Geometry: final body of the model. Coordinates: model frame, mm. A direction names the side the tool comes from. Coordinates: 2 decimals unless noted, no trailing zeros. Write each loop counter-clockwise with the first axis right and the second up, starting at its lowest first coordinate (ties: lowest second). Pieces come first, ordered by that corner, then holes. Notation, with made-up numbers: (70.5, 64) -> (124.5, 64) arc R23 cw to (124.5, 75) -> close; hole circle Ø4 at (51.5, 16). An arc over 180 degrees is marked (long way). One line per item, written item: value.
```python
from build123d import *

# Parameters (mm, degrees)
F3_D = 5.5


with BuildPart() as f1:
    # F0 (on Front) → F1 (revolve)
    with BuildSketch(Plane.XZ):
        Polygon((4, 32.5), (0, 32.5), (0, 23.5), (-2, 23.5), (-2, 18.5), (4, 18.5), align=None)
    revolve(axis=Axis((1.6395361068, 0, 0), (1, 0, 0)))

    # F3 (through all)
    with Locations(Plane(origin=(0, 0, 0), x_dir=(0, -1, 0), z_dir=(-1, 0, 0))):
        with Locations((0, 28), (28, 0), (0, -28), (-28, 0)):
            Hole(F3_D / 2)


solid = f1.part
```
(1) Line query: line 1 (Z direction, x = 2.75, y = 0); line 2 (Y direction, x = 2.2, z = 2); line 3 (X direction, y = -29, z = -6.5). Output: solid intervals per line, ascending. Write a range as [from, to].
Responses:
line 1: z = [-32.5, -30.75], [-25.25, -18.5], [18.5, 25.25], [30.75, 32.5]
line 2: y = [-32.44, -29.89], [-26.11, -18.39], [18.39, 26.11], [29.89, 32.44]
line 3: x = [0, 4]
(2) Pull-direction query (Y, two-part tool) for faces 1 (the cylindrical face through (-1, -7.1, 22.4)), 2 (the flat face through (4, 14, -14)), 3 (the cylindrical face through (2.028, -0.358, 30.727)), 4 (the cylindrical face through (2.028, 25.253, 0.121)); classes: released by +Y, released by -Y, zero draft, split by the parting line, or undercut.
Responses:
face 1: split by the parting line
face 2: zero draft
face 3: undercut
face 4: undercut
(3) Section A-A (z = 0). Return the cut outline in (x, y), then the cut area to 3 significant figures.
Responses:
outline: (-2, -23.5) -> (0, -23.5) -> (0, -25.25) -> (4, -25.25) -> (4, -18.5) -> (-2, -18.5) -> close; (-2, 18.5) -> (4, 18.5) -> (4, 25.25) -> (0, 25.25) -> (0, 23.5) -> (-2, 23.5) -> close; (0, -32.5) -> (4, -32.5) -> (4, -30.75) -> (0, -30.75) -> close; (0, 30.75) -> (4, 30.75) -> (4, 32.5) -> (0, 32.5) -> close
area: 88.0 mm2
(4) Reachability of faces 5 (the cylindrical face through (1.04, 18.06, -4.01)), 6 (the flat face through (0, 9, 22)) from +Z, -Z, +X, -X, +Y, -Y: full face, straight path, thin tool, end or side. Return the list, or none.
Responses:
face 5: +X, -X
face 6: -X
(5) First-contact query: pin 1 (7 mm diameter, centred on y = -28, z = 0, fed in from -X); pin 2 (5 mm diameter, centred on y = 0, z = 28, fed in from +X); pin 3 (3 mm diameter, centred on x = 2.5, y = 20, fed in from +Z). Flat tips, straight axial feed; report the tip coordinate or a pass-through.
Responses:
pin 1: stops at x = 0
pin 2: passes through
pin 3: stops at z = 26.72
(6) Section C-C (y = 28). Return the cut outline in (x, z).
Responses:
outline: (0, -16.5) -> (4, -16.5) -> (4, -2.75) -> (0, -2.75) -> close; (0, 2.75) -> (4, 2.75) -> (4, 16.5) -> (0, 16.5) -> close
(7) Section D-D (x = 2.15). Return the cut outline in (y, z), then the cut area to 3 significant figures.
Responses:
outline: circle Ø65 at (0, 0); hole circle Ø5.5 at (-28, 0); hole circle Ø37 at (0, 0); hole circle Ø5.5 at (0, -28); hole circle Ø5.5 at (0, 28); hole circle Ø5.5 at (28, 0)
area: 2,150 mm2
